```python
from build123d import *

# Parameters (mm, degrees)
BOSS_EXTRUDE1_DEPTH = 50
BOSS_EXTRUDE2_DEPTH = 15
BOSS_EXTRUDE3_START = 35
BOSS_EXTRUDE3_DEPTH = 15


with BuildPart() as part:
    # Sketch1 → Boss-Extrude1 (new body)
    with BuildSketch(Plane.XY):
        Polygon((30, 10), (70, 10), (90, 10), (100, 0), (0, 0), (10, 10), align=None)
    extrude(amount=BOSS_EXTRUDE1_DEPTH)

    # Sketch1<3> → Boss-Extrude2 (add)
    with BuildSketch(Plane.XY):
        with BuildLine():
            Line((70, 10), (70, 60))
            ThreePointArc((70, 60), (50, 80), (30, 60))
            Line((30, 60), (30, 10))
            Line((30, 10), (70, 10))
        make_face()
        with BuildLine():
            ThreePointArc((40, 30), (50, 20), (60, 30))
            Line((60, 30), (60, 60))
            ThreePointArc((60, 60), (50, 70), (40, 60))
            Line((40, 60), (40, 30))
        make_face(mode=Mode.SUBTRACT)
    extrude(amount=BOSS_EXTRUDE2_DEPTH)

    # Sketch1<4> → Boss-Extrude3 (add)
    with BuildSketch(Plane.XY.offset(BOSS_EXTRUDE3_START)):
        with BuildLine():
            Line((70, 10), (70, 60))
            ThreePointArc((70, 60), (50, 80), (30, 60))
            Line((30, 60), (30, 10))
            Line((30, 10), (70, 10))
        make_face()
        with BuildLine():
            ThreePointArc((40, 30), (50, 20), (60, 30))
            Line((60, 30), (60, 60))
            ThreePointArc((60, 60), (50, 70), (40, 60))
            Line((40, 60), (40, 30))
        make_face(mode=Mode.SUBTRACT)
    extrude(amount=BOSS_EXTRUDE3_DEPTH)


solid = part.part
```
Geometry check sheet. Reference: the model listing, model coordinates, mm. A direction names the side the tool comes from. Round coordinates to 2 decimals unless told otherwise and drop trailing zeros. Loops run counter-clockwise (first coordinate to the right, second up) from the corner with the lowest first, then second, coordinate; pieces in that order, holes last. Notation, with made-up numbers: (51.5, -16.75) - (83.5, -16.75) arc R16 cw to (83.5, 6.25) - close; hole circle Ø5 at (2.5, 28.25). An arc over 180 degrees is marked (long way). Write item = value, one per line. Start each with the question number.
1. Thickness scan on line 1 (Z direction, x = 61, y = 48); line 2 (X direction, y = 51, z = 11.5); line 3 (Y direction, x = 41, z = 25). Record the ranges inside material, lowest first.
2. Mould release check, pull along Z, two halves, no side actions. Record for faces 6 (the face through (58, 22, 50)), 7 (the face through (63, 45, 35)), 8 (the face through (51, 10, 25)), 9 (the face through (70, 35, 7)): released by +Z, released by -Z, zero draft, split by the parting line, or undercut.
3. Set-up check for faces 1 (the face through (30, 35, 7)), 2 (the face through (50, 20, 7)), 3 (the face through (70, 35, 42)), 4 (the face through (63, 45, 15)), 5 (the face through (50, 80, 7)): record each of +Z, -Z, +X, -X, +Y, -Y from which the full face is reachable in a straight line by a thin tool's end or side.
4. Section check D-D on y = 64. Enter the section's corners in (x, z).
5. Section check C-C on z = 10. Enter the section's corners in (x, y).
6. Section check A-A on x = 50. Enter the section's corners in (y, z), then the cut area to 3 significant figures.
7. Depth check by flat-ended pin: pin 1 (4.5 mm diameter, centred on y = 29, z = 44, fed in from -X); pin 2 (1.5 mm diameter, centred on x = 88, z = 42, fed in from +Y); pin 3 (12 mm diameter, centred on y = 41.5, z = 4, fed in from +X). Enter the tip coordinate at first touch or a pass-through.
8. Section check B-B on y = 52. Enter the section's corners in (x, z).
Working result:
q1.line_1 = 0 to 15, 35 to 50
q1.line_2 = 30 to 40, 60 to 70
q1.line_3 = 0 to 10
q2.face_6 = released by +Z
q2.face_7 = undercut
q2.face_8 = undercut
q2.face_9 = zero draft
q3.face_1 = +Z, -Z, -X, +Y
q3.face_2 = +Z, -Z
q3.face_3 = +Z, -Z, +X, +Y
q3.face_4 = +X, -X, +Y
q3.face_5 = +Z, -Z, +Y
q4.outline = (30.4, 0) - (40.83, 0) - (40.83, 15) - (30.4, 15) - close; (30.4, 35) - (40.83, 35) - (40.83, 50) - (30.4, 50) - close; (59.17, 0) - (69.6, 0) - (69.6, 15) - (59.17, 15) - close; (59.17, 35) - (69.6, 35) - (69.6, 50) - (59.17, 50) - close
q5.outline = (0, 0) - (100, 0) - (90, 10) - (70, 10) - (70, 60) arc R20 ccw to (30, 60) - (30, 10) - (10, 10) - close; hole (40, 30) arc R10 ccw to (60, 30) - (60, 60) arc R10 ccw to (40, 60) - close
q6.outline = (0, 0) - (20, 0) - (20, 15) - (10, 15) - (10, 35) - (20, 35) - (20, 50) - (0, 50) - close; (70, 0) - (80, 0) - (80, 15) - (70, 15) - close; (70, 35) - (80, 35) - (80, 50) - (70, 50) - close
q6.area = 1,100 mm^2
q7.pin_1 = 30
q7.pin_2 = 10
q7.pin_3 = 70
q8.outline = (30, 0) - (40, 0) - (40, 15) - (30, 15) - close; (30, 35) - (40, 35) - (40, 50) - (30, 50) - close; (60, 0) - (70, 0) - (70, 15) - (60, 15) - close; (60, 35) - (70, 35) - (70, 50) - (60, 50) - close
